For this review, take the finished solid that the model builds, in its own axes (mm). A direction names the side the tool comes from. Round coordinates to 2 decimals unless told otherwise and drop trailing zeros. Order: outer loops, then holes, each group sorted by start corner. A loop starts at its lowest first (then second) coordinate and runs counter-clockwise, first axis right, second up.
from build123d import *

# Parameters (mm, degrees)
YAW_PLATFORM_START                     = 72
YAW_PLATFORM_PROFILE_R                 = 44
YAW_PLATFORM_DEPTH                     = 5
PRINTED_HOLLOW_YAW_SPINDLE_START       = 43
PRINTED_HOLLOW_YAW_SPINDLE_PROFILE_R   = 3.95
PRINTED_HOLLOW_YAW_SPINDLE_PROFILE_R_2 = 1.75
PRINTED_HOLLOW_YAW_SPINDLE_DEPTH       = 29
INNER_RACE_LOAD_SHOULDER_START         = 70
INNER_RACE_LOAD_SHOULDER_PROFILE_R     = 6
INNER_RACE_LOAD_SHOULDER_PROFILE_R_2   = 1.75
INNER_RACE_LOAD_SHOULDER_DEPTH         = 2
D_FLAT_ON_SPINDLE_END_START            = 43
D_FLAT_DRIVE_KEY_PROFILE_W             = 3
D_FLAT_DRIVE_KEY_PROFILE_H             = 10
D_FLAT_ON_SPINDLE_END_DEPTH            = 5
SHOULDER_MOUNT_PLATE_PROFILE_W         = 66
SHOULDER_MOUNT_PLATE_PROFILE_H         = 68
SHOULDER_MOUNT_PLATE_DEPTH             = 4
MG996_BODY_WINDOW_START                = -5
MG996_BODY_WINDOW_PROFILE_W            = 41.7
MG996_BODY_WINDOW_PROFILE_H            = 20.7
MG996_BODY_WINDOW_DEPTH                = 162.869372409
MG996_TAB_MOUNTS_START                 = -50
MG996_TAB_MOUNTS_PROFILE_R             = 1.9
MG996_TAB_MOUNTS_DEPTH                 = 207.869372409
PASSIVE_SHOULDER_STANDOFFS_START       = -50
PASSIVE_SHOULDER_STANDOFFS_PROFILE_R   = 1.6
PASSIVE_SHOULDER_STANDOFFS_DEPTH       = 207.869372409
UPRIGHT_RIB_START                      = -8
UPRIGHT_RIB_PROFILE_W                  = 7
UPRIGHT_RIB_PROFILE_H                  = 31
UPRIGHT_RIB_DEPTH                      = 12


with BuildPart() as part:
    # Yaw_platform_profile → Yaw_platform (new body)
    with BuildSketch(Plane(origin=(0, 0, 0), x_dir=(1, 0, 0), z_dir=(0, 1, 0)).offset(YAW_PLATFORM_START)):
        with Locations(Location((0, 0, 0), (0, 0, 270))):
            Circle(YAW_PLATFORM_PROFILE_R)
    extrude(amount=YAW_PLATFORM_DEPTH)

    # Printed_hollow_yaw_spindle_profile → Printed_hollow_yaw_spindle (add)
    with BuildSketch(Plane(origin=(0, 0, 0), x_dir=(1, 0, 0), z_dir=(0, 1, 0)).offset(PRINTED_HOLLOW_YAW_SPINDLE_START)):
        with Locations(Location((0, 0, 0), (0, 0, 90))):
            Circle(PRINTED_HOLLOW_YAW_SPINDLE_PROFILE_R)
        with Locations(Location((0, 0, 0), (0, 0, 90))):
            Circle(PRINTED_HOLLOW_YAW_SPINDLE_PROFILE_R_2, mode=Mode.SUBTRACT)
    extrude(amount=PRINTED_HOLLOW_YAW_SPINDLE_DEPTH)

    # Inner_race_load_shoulder_profile → Inner_race_load_shoulder (add)
    with BuildSketch(Plane(origin=(0, 0, 0), x_dir=(1, 0, 0), z_dir=(0, 1, 0)).offset(INNER_RACE_LOAD_SHOULDER_START)):
        with Locations(Location((0, 0, 0), (0, 0, 270))):
            Circle(INNER_RACE_LOAD_SHOULDER_PROFILE_R)
        with Locations(Location((0, 0, 0), (0, 0, 90))):
            Circle(INNER_RACE_LOAD_SHOULDER_PROFILE_R_2, mode=Mode.SUBTRACT)
    extrude(amount=INNER_RACE_LOAD_SHOULDER_DEPTH)

    # D_flat_drive_key_profile → D_flat_on_spindle_end (cut)
    with BuildSketch(Plane(origin=(0, 0, 0), x_dir=(1, 0, 0), z_dir=(0, 1, 0)).offset(D_FLAT_ON_SPINDLE_END_START)):
        with Locations((4.5, 0)):
            Rectangle(D_FLAT_DRIVE_KEY_PROFILE_W, D_FLAT_DRIVE_KEY_PROFILE_H)
    extrude(amount=D_FLAT_ON_SPINDLE_END_DEPTH, mode=Mode.SUBTRACT)

    # Shoulder_mount_plate_profile → Shoulder_mount_plate (add)
    with BuildSketch(Plane.XY):
        with Locations((10, 110)):
            Rectangle(SHOULDER_MOUNT_PLATE_PROFILE_W, SHOULDER_MOUNT_PLATE_PROFILE_H)
    extrude(amount=SHOULDER_MOUNT_PLATE_DEPTH)

    # MG996_body_window_profile → MG996_body_window (cut, through all)
    with BuildSketch(Plane.XY.offset(MG996_BODY_WINDOW_START)):
        with Locations((10.35, 122)):
            Rectangle(MG996_BODY_WINDOW_PROFILE_W, MG996_BODY_WINDOW_PROFILE_H)
    extrude(amount=MG996_BODY_WINDOW_DEPTH, mode=Mode.SUBTRACT)

    # MG996_tab_mounts_profile → MG996_tab_mounts (cut, through all)
    with BuildSketch(Plane.XY.offset(MG996_TAB_MOUNTS_START)):
        with Locations(Location((-13, 117, 0), (0, 0, 180))):
            Circle(MG996_TAB_MOUNTS_PROFILE_R)
        with Locations(Location((-13, 127, 0), (0, 0, 180))):
            Circle(MG996_TAB_MOUNTS_PROFILE_R)
        with Locations(Location((34, 117, 0), (0, 0, 180))):
            Circle(MG996_TAB_MOUNTS_PROFILE_R)
        with Locations(Location((34, 127, 0), (0, 0, 180))):
            Circle(MG996_TAB_MOUNTS_PROFILE_R)
    extrude(amount=MG996_TAB_MOUNTS_DEPTH, mode=Mode.SUBTRACT)

    # Passive_shoulder_standoffs_profile → Passive_shoulder_standoffs (cut, through all)
    with BuildSketch(Plane.XY.offset(PASSIVE_SHOULDER_STANDOFFS_START)):
        with Locations(Location((36, 104, 0), (0, 0, 180))):
            Circle(PASSIVE_SHOULDER_STANDOFFS_PROFILE_R)
        with Locations(Location((36, 140, 0), (0, 0, 180))):
            Circle(PASSIVE_SHOULDER_STANDOFFS_PROFILE_R)
    extrude(amount=PASSIVE_SHOULDER_STANDOFFS_DEPTH, mode=Mode.SUBTRACT)

    # Upright_rib_profile → Upright_rib (add)
    with BuildSketch(Plane.XY.offset(UPRIGHT_RIB_START)):
        with Locations((-19.5, 92.5)):
            Rectangle(UPRIGHT_RIB_PROFILE_W, UPRIGHT_RIB_PROFILE_H)
    extrude(amount=UPRIGHT_RIB_DEPTH)


solid = part.part
(1) Draft analysis for pull direction X (two halves, no side actions). For faces 5 (the face through (-23, 103, -1)), 6 (the face through (31.2, 122, 2)), 7 (the face through (10, 111, 4)), state which applies: pulls with the +X half, pulls with the -X half, needs draft (parallel to the pull), parting line crosses it, or undercut.
(2) Add section B-B on x = 0. Give the boundary of the cut face in (y, z), plus the area to 3 significant figures.
(3) Wall thickness on L1, parallel to Y at x = 34, z = 3; L2, parallel to X at y = 127, z = 2.9; L3, parallel to Y at x = 36, z = 2: over which ranges is each line inside the solid? List them lowest first.
(4) Clearance check with flat-ended pins moving along their axes: P1, Ø3.5, axis at y = 124.5, z = 0, coming from the -X side; P2, Ø6, axis at x = 34, y = 127, coming from the +Z side; P3, Ø6, axis at x = -29, z = 18.5, coming from the +Y side. State where each tip first meets the part, or that it passes through.
(5) Add section D-D on x = -13. Give the boundary of the cut face in (y, z), plus the area to 3 significant figures.
(6) Tool access review of faces 1 (the face through (1.802, 70.986, 5.723)), 2 (the face through (-20, 93, -8)), 3 (the face through (-16, 92, -4)), 4 (the face through (-10.5, 122, 2)): name each direction out of +Z, -Z, +X, -X, +Y, -Y from which nothing blocks a thin tool from reaching the whole face with its end or side.
(7) Add section C-C on y = 127. Give the boundary of the cut face in (x, z), plus the area to 3 significant figures.
(8) Add section A-A on y = 113.5. Give the boundary of the cut face in (x, z).
Here are the results:
1. face 5: pulls with the -X half
1. face 6: undercut
1. face 7: needs draft
2. outline: (43, -3.95) - (70, -3.95) - (70, -6) - (72, -6) - (72, -44) - (77, -44) - (77, 0) - (111.65, 0) - (111.65, 4) - (77, 4) - (77, 44) - (72, 44) - (72, 6) - (70, 6) - (70, 3.95) - (43, 3.95) - (43, 1.75) - (72, 1.75) - (72, -1.75) - (43, -1.75) - close; (132.35, 0) - (144, 0) - (144, 4) - (132.35, 4) - close
2. area: 761 mm2
3. L1: y = 72 to 115.1, 118.9 to 125.1, 128.9 to 144
3. L2: x = -23 to -14.9, -11.1 to -10.5, 31.2 to 32.1, 35.9 to 43
3. L3: y = 72 to 102.4, 105.6 to 138.4, 141.6 to 144
4. P1: stops at x = -23
4. P2: stops at z = 4
4. P3: stops at y = 77
5. outline: (72, -42.04) - (77, -42.04) - (77, 0) - (115.1, 0) - (115.1, 4) - (77, 4) - (77, 42.04) - (72, 42.04) - close; (118.9, 0) - (125.1, 0) - (125.1, 4) - (118.9, 4) - close; (128.9, 0) - (144, 0) - (144, 4) - (128.9, 4) - close
5. area: 658 mm2
6. face 1: -Y
6. face 2: -Z, +X, -X, +Y
6. face 3: -Z, +X, +Y
6. face 4: +Z, -Z
7. outline: (-23, 0) - (-14.9, 0) - (-14.9, 4) - (-23, 4) - close; (-11.1, 0) - (-10.5, 0) - (-10.5, 4) - (-11.1, 4) - close; (31.2, 0) - (32.1, 0) - (32.1, 4) - (31.2, 4) - close; (35.9, 0) - (43, 0) - (43, 4) - (35.9, 4) - close
7. area: 66.8 mm2
8. outline: (-23, 0) - (-10.5, 0) - (-10.5, 4) - (-23, 4) - close; (31.2, 0) - (43, 0) - (43, 4) - (31.2, 4) - close
